Read the model definition and answer for the solid it produces. Units are mm, in the model's axes. Face numbers are marked on the shaded views. A direction names the side the tool comes from. Coordinates: 2 decimals unless noted, no trailing zeros. Order: outer loops, then holes, each group sorted by start corner. A loop starts at its lowest first (then second) coordinate and runs counter-clockwise, first axis right, second up. Notation, with made-up numbers: M 80.25,68.25 L 120.25,68.25 A14 cw 120.25,82.25 Z; hole C 89,18 d4. An arc over 180 degrees is marked long. Use a Markdown table: item, result. Add a question column.
1) Find the intervals of material crossed by probe 1 along X at (y, z) = (12, -4); probe 2 along X at (y, z) = (-11.5, -5); probe 3 along Z at (x, y) = (-7, -18.5), in increasing order. Write a range as [from, to].
2) Find section A-A on y = -12.7. Write down the section's boundary in (x, z).
3) Find section B-B on x = 24.5. Write down the section's boundary in (y, z).
4) Each of these flat-tipped pins is pushed along its axis until it touches: pin 1 Ø5 at (y, z) = (15.5, -17.5) entering from +X; pin 2 Ø1 at (y, z) = (-5, -50.5) entering from +X; pin 3 Ø10.5 at (x, y) = (-75.36, 12.7) entering from -Z. Where does it stop, or does it pass through?
5) Find section D-D on y = 5. Write down the section's boundary in (x, z), plus the area to 3 significant figures.
6) The mould has two halves that part along X. Classify the marked faces 1, 2 and 3: released by +X, released by -X, zero draft, split by the parting line, or undercut.
7) For the marked faces 4, 5 and 6, determine the directions among +Z, -Z, +X, -X, +Y, -Y from which every point of the face is accessible in a straight line to the end or side of a thin tool.
8) Find section C-C on z = -34.5. Write down the section's boundary in (x, y), plus the area to 3 significant figures.
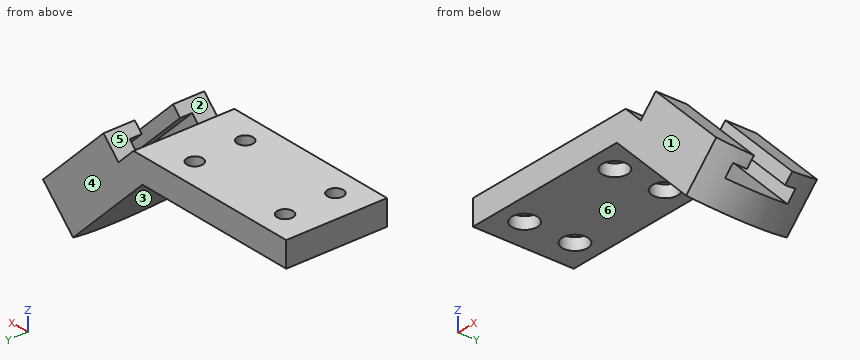
from build123d import *

# Parameters (mm, degrees)
F0_W           = 91.11234
F0_H           = 50.8
F3_DEPTH       = 12.7
F4_DEPTH       = 12.7
F6_DEPTH       = 82.805
F7_DEPTH       = 12.7
F9_D           = 7.9248
F9_CBORE_D     = 12.7
F9_CBORE_DEPTH = 6.096


with BuildPart() as f3:
    # F0 (on Top) → F3 (new body)
    with BuildSketch(Plane.XY):
        with Locations((-45.55617, 0)):
            Rectangle(F0_W, F0_H)
    extrude(amount=-F3_DEPTH)

    # F2 (on line) → F4 (join, symmetric)
    with BuildSketch(Plane(origin=(0, 0, 0), x_dir=(0.7071067812, 0, -0.7071067812), z_dir=(-0.7071067812, 0, -0.7071067812))):
        with BuildLine():
            Line((63.7370183547, 25.4), (0, 25.4))
            Line((0, 25.4), (0, -25.4))
            Line((0, -25.4), (63.7370183547, -25.4))
            ThreePointArc((63.7370183547, -25.4), (70.104, 0), (63.7370183547, 25.4))
        make_face()
    extrude(amount=F4_DEPTH, both=True)

    # F5 (on face) → F6 (cut, through all)
    with BuildSketch(Plane(origin=(0, 0, 0), x_dir=(0, -1, 0), z_dir=(-0.7071067812, 0, 0.7071067812))):
        Polygon((-15.748, 6.6890539291), (-15.748, 0), (15.748, 0), (15.748, 6.6890539291), (9.6519063121, 6.6890539291), (9.6519063121, 12.7), (-9.6519063121, 12.7), (-9.6519063121, 6.6890539291), align=None)
    extrude(amount=-F6_DEPTH, mode=Mode.SUBTRACT)

    # F5 (on face) → F7 (cut)
    with BuildSketch(Plane(origin=(0, 0, 0), x_dir=(0, -1, 0), z_dir=(-0.7071067812, 0, 0.7071067812))):
        Polygon((-25.4, 12.7), (-25.4, 0), (-15.748, 0), (-15.748, 6.6890539291), (-9.6519063121, 6.6890539291), (-9.6519063121, 12.7), align=None)
        Polygon((15.748, 6.6890539291), (15.748, 0), (25.4, 0), (25.4, 12.7), (9.6519063121, 12.7), (9.6519063121, 6.6890539291), align=None)
    extrude(amount=-F7_DEPTH, mode=Mode.SUBTRACT)

    # F9 (through all)
    with Locations(Plane(origin=(0, 0, -12.7), x_dir=(1, 0, 0), z_dir=(0, 0, -1))):
        with Locations((-75.36434, 12.7), (-75.36434, -12.7), (-21.51634, 12.7), (-21.51634, -12.7)):
            CounterBoreHole(F9_D / 2, F9_CBORE_D / 2, F9_CBORE_DEPTH)


solid = f3.part
Check result:
| question | item | result |
|---|---|---|
| 1 | probe 1 | x = [-91.11, -79.26], [-71.46, -25.42], [-17.62, 4], [13.96, 21.96] |
| 1 | probe 2 | x = [-91.11, -79.14], [-71.59, -25.29], [-17.74, 5], [14.46, 22.96] |
| 1 | probe 3 | z = [-12.7, 0] |
| 2 | outline | M -91.11,-12.7 L -81.71,-12.7 L -81.71,-6.6 L -79.33,-6.6 L -79.33,0 L -91.11,0 Z; M -71.4,-6.6 L -69.01,-6.6 L -69.01,-12.7 L -27.87,-12.7 L -27.87,-6.6 L -25.48,-6.6 L -25.48,0 L -71.4,0 Z; M -17.55,-6.6 L -15.17,-6.6 L -15.17,-12.7 L -5.26,-12.7 L 39.52,-57.48 L 48.5,-48.5 L 0,0 L -17.55,0 Z; M 13.71,-4.25 L 53.23,-43.77 L 57.48,-39.52 L 17.96,0 Z |
| 3 | outline | M -25.4,-42.46 L 25.4,-42.46 L 25.4,-6.54 L 9.65,-6.54 L 9.65,-15.04 L 15.75,-15.04 L 15.75,-24.5 L -15.75,-24.5 L -15.75,-15.04 L -9.65,-15.04 L -9.65,-6.54 L -25.4,-6.54 Z |
| 4 | pin 1 | stops at x = 37.96 |
| 4 | pin 2 | stops at x = 48.82 |
| 4 | pin 3 | stops at z = -6.6 |
| 5 | outline | M -91.11,-12.7 L -5.26,-12.7 L 40.43,-58.39 L 49.41,-49.41 L 0,0 L -91.11,0 Z |
| 5 | area | 1,980 mm2 |
| 6 | face 1 | zero draft |
| 6 | face 2 | undercut |
| 6 | face 3 | released by -X |
| 7 | face 4 | +Z, -Z, +X, -X, +Y |
| 7 | face 5 | +Z, +Y, -Y |
| 7 | face 6 | -Z, -X, +Y, -Y |
| 8 | outline | M 16.54,-25.4 L 52.46,-25.4 L 52.46,-9.65 L 43.96,-9.65 L 43.96,-15.75 L 34.5,-15.75 L 34.5,15.75 L 43.96,15.75 L 43.96,9.65 L 52.46,9.65 L 52.46,25.4 L 16.54,25.4 Z |
| 8 | area | 1,360 mm2 |
